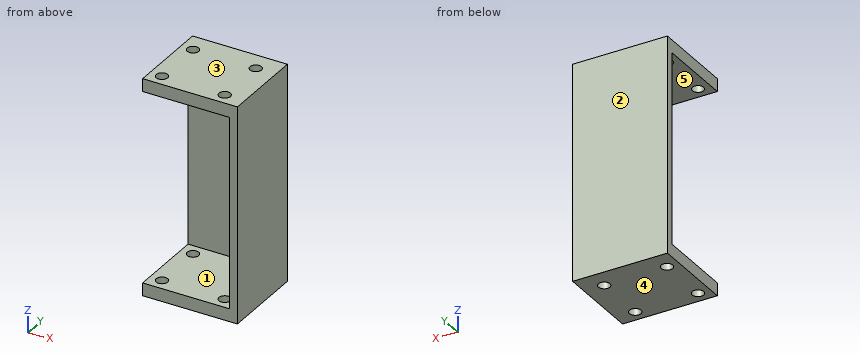
from build123d import *

# Parameters (mm, degrees)
SKETCH1_W           = 34
SKETCH1_H           = 30
SKETCH1_R           = 2.25
BOSS_EXTRUDE1_DEPTH = 5
SKETCH2_W           = 5
SKETCH2_H           = 30
BOSS_EXTRUDE2_DEPTH = 15
SKETCH4_W           = 5
SKETCH4_H           = 30
BOSS_EXTRUDE3_DEPTH = 25
SKETCH5_R           = 2.5
CUT_EXTRUDE1_DEPTH  = 25
SKETCH6_W           = 15
SKETCH6_H           = 30
CUT_EXTRUDE2_DEPTH  = 66
SKETCH7_W           = 34
SKETCH7_H           = 30
SKETCH7_R           = 2.25
BOSS_EXTRUDE4_DEPTH = 79.5
SKETCH8_W           = 34
SKETCH8_H           = 74.5
CUT_EXTRUDE3_DEPTH  = 30
BOSS_EXTRUDE6_DEPTH = 84.5


with BuildPart() as part:
    # Sketch1 → Boss-Extrude1 (new body)
    with BuildSketch(Plane.XY):
        with Locations((17, 15)):
            Rectangle(SKETCH1_W, SKETCH1_H)
        with Locations((4.75, 25.25)):
            Circle(SKETCH1_R, mode=Mode.SUBTRACT)
        with Locations((29.25, 25.25)):
            Circle(SKETCH1_R, mode=Mode.SUBTRACT)
        with Locations((29.25, 4.75)):
            Circle(SKETCH1_R, mode=Mode.SUBTRACT)
        with Locations((4.75, 4.75)):
            Circle(SKETCH1_R, mode=Mode.SUBTRACT)
    extrude(amount=BOSS_EXTRUDE1_DEPTH)

    # Sketch2 → Boss-Extrude2 (add)
    with BuildSketch(Plane.ZY):
        with Locations((2.5, 15)):
            Rectangle(SKETCH2_W, SKETCH2_H)
    extrude(amount=BOSS_EXTRUDE2_DEPTH)

    # Sketch4 → Boss-Extrude3 (add)
    with BuildSketch(Plane.XY.offset(5)):
        with Locations((-12.5, 15)):
            Rectangle(SKETCH4_W, SKETCH4_H)
    extrude(amount=BOSS_EXTRUDE3_DEPTH)

    # Sketch5 → Cut-Extrude1 (cut)
    with BuildSketch(Plane(origin=(-10, 0, 0), x_dir=(0, 0, -1), z_dir=(1, 0, 0))):
        with Locations((-24, 15)):
            Circle(SKETCH5_R)
        with Locations((-10, 15)):
            Circle(SKETCH5_R)
    extrude(amount=-CUT_EXTRUDE1_DEPTH, mode=Mode.SUBTRACT)

    # Sketch6 → Cut-Extrude2 (cut)
    with BuildSketch(Plane(origin=(0, 30, 0), x_dir=(1, 0, 0), z_dir=(0, 1, 0))):
        with Locations((-7.5, -15)):
            Rectangle(SKETCH6_W, SKETCH6_H)
    extrude(amount=-CUT_EXTRUDE2_DEPTH, mode=Mode.SUBTRACT)

    # Sketch7 → Boss-Extrude4 (add)
    with BuildSketch(Plane.XY.offset(5)):
        with Locations((17, 15)):
            Rectangle(SKETCH7_W, SKETCH7_H)
        with Locations((4.75, 25.25)):
            Circle(SKETCH7_R, mode=Mode.SUBTRACT)
        with Locations((29.25, 25.25)):
            Circle(SKETCH7_R, mode=Mode.SUBTRACT)
        with Locations((29.25, 4.75)):
            Circle(SKETCH7_R, mode=Mode.SUBTRACT)
        with Locations((4.75, 4.75)):
            Circle(SKETCH7_R, mode=Mode.SUBTRACT)
    extrude(amount=BOSS_EXTRUDE4_DEPTH)

    # Sketch8 → Cut-Extrude3 (cut)
    with BuildSketch(Plane(origin=(0, 30, 0), x_dir=(1, 0, 0), z_dir=(0, 1, 0))):
        with Locations((17, -42.25)):
            Rectangle(SKETCH8_W, SKETCH8_H)
    extrude(amount=-CUT_EXTRUDE3_DEPTH, mode=Mode.SUBTRACT)


with BuildPart() as cut_extrude3_piece_1:
    # of the separate pieces the step leaves, piece 1, a body of its own (cut_extrude3_pieces)
    add(part.part.solids().sort_by_distance((34, 0, 0))[0])



with BuildPart() as cut_extrude3_piece_2:
    # of the separate pieces the step leaves, piece 2, a body of its own (cut_extrude3_pieces)
    add(part.part.solids().sort_by_distance((34, 0, 79.5))[0])


with BuildPart() as cut_extrude3_piece_1_1:
    add(cut_extrude3_piece_1.part)

    add(cut_extrude3_piece_2.part)  # Boss-Extrude6 merges Cut-Extrude3 piece 2
    # Sketch11 → Boss-Extrude6 (add)
    with BuildSketch(Plane(origin=(0, 0, 0), x_dir=(-1, 0, 0), z_dir=(0, 0, -1))):
        Polygon((0, 30), (0, 33), (-37, 33), (-37, 0), (-34, 0), (-34, 30), align=None)
    extrude(amount=-BOSS_EXTRUDE6_DEPTH)


solid = cut_extrude3_piece_1_1.part
For this review, take the finished solid that the model builds, in its own axes (mm). Face numbers are marked on the shaded views. A direction names the side the tool comes from. Round coordinates to 2 decimals unless told otherwise and drop trailing zeros. Order: outer loops, then holes, each group sorted by start corner. A loop starts at its lowest first (then second) coordinate and runs counter-clockwise, first axis right, second up. Notation, with made-up numbers: M 1.25,-1.75 L 32.25,-1.75 A24 ccw 32.25,10.25 Z; hole C 79.25,9.25 d3. An arc over 180 degrees is marked long. Write each question's results on one line, items separated by ' | '. Start each with the question number.
1. Add section A-A (y = 4.75). State the section outline as (x, z) points.
2. Add section B-B (x = 29.25). State the section outline as (y, z) points, then the cut area to 4 significant figures.
3. Clearance check with flat-ended pins moving along their axes: pin 1 Ø5 at (x, z) = (15, 68) entering from -Y; pin 2 Ø15 at (y, z) = (19.5, 50) entering from -X. State where each tip first meets the part, or that it passes through.
4. To check wall thickness, follow L1, parallel to X at y = 4.75, z = 3.9; L2, parallel to Y at x = 29.25, z = 81.3; L3, parallel to Z at x = 15.5, y = 22.5. State the ranges of each line that lie inside material, in increasing order. Write a range as [from, to].
5. Add section D-D (z = 38.5). State the section outline as (x, y) points.
6. Add section C-C (y = 10.5). State the section outline as (x, z) points.
7. Tool access review of the marked faces 1 and 2: name each direction out of +Z, -Z, +X, -X, +Y, -Y from which nothing blocks a thin tool from reaching the whole face with its end or side.
8. Draft analysis for pull direction Z (two halves, no side actions). For the marked faces 3, 4 and 5, state which applies: pulls with the +Z half, pulls with the -Z half, needs draft (parallel to the pull), parting line crosses it, or undercut.
Output values:
1) outline: M 0,0 L 2.5,0 L 2.5,5 L 0,5 Z; M 0,79.5 L 2.5,79.5 L 2.5,84.5 L 0,84.5 Z; M 7,0 L 27,0 L 27,5 L 7,5 Z; M 7,79.5 L 27,79.5 L 27,84.5 L 7,84.5 Z; M 31.5,0 L 37,0 L 37,84.5 L 31.5,84.5 L 31.5,79.5 L 34,79.5 L 34,5 L 31.5,5 Z
2) outline: M 0,0 L 2.5,0 L 2.5,5 L 0,5 Z; M 0,79.5 L 2.5,79.5 L 2.5,84.5 L 0,84.5 Z; M 7,0 L 23,0 L 23,5 L 7,5 Z; M 7,79.5 L 23,79.5 L 23,84.5 L 7,84.5 Z; M 27.5,0 L 33,0 L 33,84.5 L 27.5,84.5 L 27.5,79.5 L 30,79.5 L 30,5 L 27.5,5 Z | area: 463.5 mm^2
3) pin 1: y = 30 | pin 2: x = 34
4) L1: [0, 2.5], [7, 27], [31.5, 37] | L2: [0, 2.5], [7, 23], [27.5, 33] | L3: [0, 5], [79.5, 84.5]
5) outline: M 0,30 L 34,30 L 34,0 L 37,0 L 37,33 L 0,33 Z
6) outline: M 0,0 L 37,0 L 37,84.5 L 0,84.5 L 0,79.5 L 34,79.5 L 34,5 L 0,5 Z
7) face 1: -X, -Y | face 2: +Z, -Z, +X, -X, +Y
8) face 3: pulls with the +Z half | face 4: pulls with the -Z half | face 5: undercut
